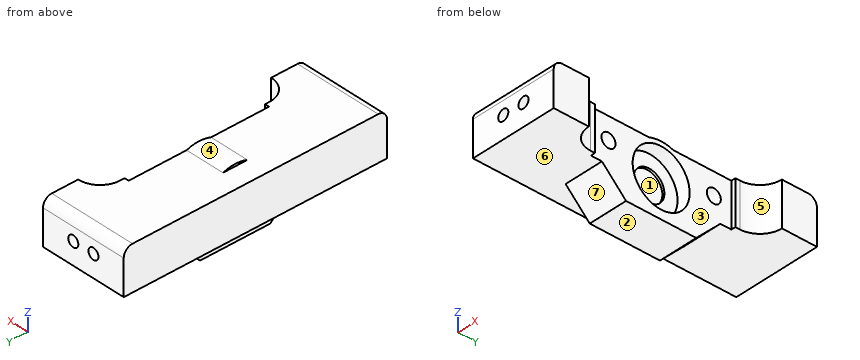
```python
from build123d import *

# Parameters (mm, degrees)
BOX035_W          = 5
BOX035_H          = 60
BOX035_DEPTH      = 10
BOX033_W          = 5
BOX033_H          = 8
BOX033_DEPTH      = 10
FILLET011_R       = 2
BOX034_W          = 5
BOX034_H          = 8
BOX034_DEPTH      = 10
FILLET012_R       = 2
BOX030_W          = 1
BOX030_H          = 32
BOX030_DEPTH      = 22
CYLINDER072_R     = 1.6
CYLINDER072_DEPTH = 10
CYLINDER071_R     = 1.6
CYLINDER071_DEPTH = 10
CYLINDER062_R     = 1.25
CYLINDER062_DEPTH = 10
CYLINDER060_R     = 1.25
CYLINDER060_DEPTH = 10
CYLINDER061_R     = 1.25
CYLINDER061_DEPTH = 10
CYLINDER059_R     = 1.25
CYLINDER059_DEPTH = 10
CYLINDER047_R     = 3.5
CYLINDER047_DEPTH = 4
CYLINDER045_R     = 6.5
CYLINDER045_DEPTH = 4
BOX031_W          = 15
BOX031_H          = 16
BOX031_DEPTH      = 5.5
CYLINDER046_R     = 8
CYLINDER046_DEPTH = 10
BOX021_W          = 10
BOX021_H          = 60
BOX021_DEPTH      = 10
BOX032_W          = 5
BOX032_H          = 60
BOX032_DEPTH      = 10
FILLET010_R       = 2
CHAMFER002_SIZE   = 5.49
FILLET013_R       = 4.99


with BuildPart() as cube014:
    # Box035 → Box035 (new body)
    with BuildSketch(Plane(origin=(75, 1, -1), x_dir=(1, 0, 0), z_dir=(0, 0, 1))):
        with Locations((2.5, 30)):
            Rectangle(BOX035_W, BOX035_H)
    extrude(amount=BOX035_DEPTH)


with BuildPart() as fillet011:
    # Box033 → Box033 (new body)
    with BuildSketch(Plane(origin=(90, 1, 9), x_dir=(1, 0, 0), z_dir=(0, 0, 1))):
        with Locations((2.5, 4)):
            Rectangle(BOX033_W, BOX033_H)
    extrude(amount=BOX033_DEPTH)

    # Fillet011
    fillet011_edges = [fillet011.edges().sort_by_distance(p)[0] for p in [
        (92.5, 1, 19),
    ]]
    fillet(fillet011_edges, radius=FILLET011_R)


with BuildPart() as fillet012:
    # Box034 → Box034 (new body)
    with BuildSketch(Plane(origin=(90, 53, 9), x_dir=(1, 0, 0), z_dir=(0, 0, 1))):
        with Locations((2.5, 4)):
            Rectangle(BOX034_W, BOX034_H)
    extrude(amount=BOX034_DEPTH)

    # Fillet012
    fillet012_edges = [fillet012.edges().sort_by_distance(p)[0] for p in [
        (92.5, 61, 19),
    ]]
    fillet(fillet012_edges, radius=FILLET012_R)


with BuildPart() as cube009:
    # Box030 → Box030 (new body)
    with BuildSketch(Plane(origin=(89, 15, 2), x_dir=(1, 0, 0), z_dir=(0, 0, 1))):
        with Locations((0.5, 16)):
            Rectangle(BOX030_W, BOX030_H)
    extrude(amount=BOX030_DEPTH)


with BuildPart() as cylinder072:
    # Cylinder072 → Cylinder072 (new body)
    with BuildSketch(Plane(origin=(80, 43, 14), x_dir=(0, 0, -1), z_dir=(1, 0, 0))):
        Circle(CYLINDER072_R)
    extrude(amount=CYLINDER072_DEPTH)


with BuildPart() as fusion068:
    # Cylinder071 → Cylinder071 (new body)
    with BuildSketch(Plane(origin=(80, 19, 14), x_dir=(0, 0, -1), z_dir=(1, 0, 0))):
        Circle(CYLINDER071_R)
    extrude(amount=CYLINDER071_DEPTH)

    # Fusion068: union Cylinder072
    add(cylinder072.part)


with BuildPart() as cylinder062:
    # Cylinder062 → Cylinder062 (new body)
    with BuildSketch(Plane(origin=(87.5, 61, 14), x_dir=(1, 0, 0), z_dir=(0, -1, 0))):
        Circle(CYLINDER062_R)
    extrude(amount=CYLINDER062_DEPTH)


with BuildPart() as fusion046:
    # Cylinder060 → Cylinder060 (new body)
    with BuildSketch(Plane(origin=(87.5, 11, 14), x_dir=(1, 0, 0), z_dir=(0, -1, 0))):
        Circle(CYLINDER060_R)
    extrude(amount=CYLINDER060_DEPTH)

    # Fusion046: union Cylinder062
    add(cylinder062.part)


with BuildPart() as cylinder061:
    # Cylinder061 → Cylinder061 (new body)
    with BuildSketch(Plane(origin=(82.5, 61, 14), x_dir=(1, 0, 0), z_dir=(0, -1, 0))):
        Circle(CYLINDER061_R)
    extrude(amount=CYLINDER061_DEPTH)


with BuildPart() as fusion048:
    # Cylinder059 → Cylinder059 (new body)
    with BuildSketch(Plane(origin=(82.5, 11, 14), x_dir=(1, 0, 0), z_dir=(0, -1, 0))):
        Circle(CYLINDER059_R)
    extrude(amount=CYLINDER059_DEPTH)

    # Fusion045: union Cylinder061
    add(cylinder061.part)

    # Fusion048: union Fusion046
    add(fusion046.part)


with BuildPart() as cylinder047:
    # Cylinder047 → Cylinder047 (new body)
    with BuildSketch(Plane(origin=(89.5, 31, 10), x_dir=(0, 0, -1), z_dir=(1, 0, 0))):
        Circle(CYLINDER047_R)
    extrude(amount=CYLINDER047_DEPTH)


with BuildPart() as fusion037:
    # Cylinder045 → Cylinder045 (new body)
    with BuildSketch(Plane(origin=(90, 31, 10), x_dir=(0, 0, -1), z_dir=(1, 0, 0))):
        Circle(CYLINDER045_R)
    extrude(amount=CYLINDER045_DEPTH)

    # Fusion037: union Cylinder047
    add(cylinder047.part)


with BuildPart() as fusion037_1:
    # Fusion037 placement: moved
    add(fusion037.part.moved(Location((-4, 0, 2))))


with BuildPart() as cube010:
    # Box031 → Box031 (new body)
    with BuildSketch(Plane(origin=(75, 23, 3.5), x_dir=(1, 0, 0), z_dir=(0, 0, 1))):
        with Locations((7.5, 8)):
            Rectangle(BOX031_W, BOX031_H)
    extrude(amount=BOX031_DEPTH)


with BuildPart() as cylinder046:
    # Cylinder046 → Cylinder046 (new body)
    with BuildSketch(Plane(origin=(80, 31, 11.5), x_dir=(0, 0, -1), z_dir=(1, 0, 0))):
        Circle(CYLINDER046_R)
    extrude(amount=CYLINDER046_DEPTH)


with BuildPart() as fusion038:
    # Box021 → Box021 (new body)
    with BuildSketch(Plane(origin=(80, 1, 9), x_dir=(1, 0, 0), z_dir=(0, 0, 1))):
        with Locations((5, 30)):
            Rectangle(BOX021_W, BOX021_H)
    extrude(amount=BOX021_DEPTH)

    # Fusion038: union Cylinder046
    add(cylinder046.part)


with BuildPart() as front_threaded_bar_support:
    # Box032 → Box032 (new body)
    with BuildSketch(Plane(origin=(75, 1, 9), x_dir=(1, 0, 0), z_dir=(0, 0, 1))):
        with Locations((2.5, 30)):
            Rectangle(BOX032_W, BOX032_H)
    extrude(amount=BOX032_DEPTH)

    # Fusion069: union Cube010, Fusion038
    add(cube010.part)
    add(fusion038.part)

    # Cut037: cut Fusion037
    add(fusion037_1.part, mode=Mode.SUBTRACT)

    # Cut038: cut Fusion048
    add(fusion048.part, mode=Mode.SUBTRACT)

    # Cut039: cut Fusion068
    add(fusion068.part, mode=Mode.SUBTRACT)

    # Cut040: cut Cube009
    add(cube009.part, mode=Mode.SUBTRACT)

    # Fillet010
    fillet010_edges = [front_threaded_bar_support.edges().sort_by_distance(p)[0] for p in [
        (82.5, 1, 19),
        (82.5, 61, 19),
    ]]
    fillet(fillet010_edges, radius=FILLET010_R)

    # Chamfer002
    chamfer002_edges = [front_threaded_bar_support.edges().sort_by_distance(p)[0] for p in [
        (82, 23, 9),
        (82, 39, 9),
    ]]
    chamfer(chamfer002_edges, length=CHAMFER002_SIZE)

    # Fusion070: union Fillet011, Fillet012
    add(fillet011.part)
    add(fillet012.part)

    # Fillet013
    fillet013_edges = [front_threaded_bar_support.edges().sort_by_distance(p)[0] for p in [
        (90, 53, 14),
        (90, 9, 14),
    ]]
    fillet(fillet013_edges, radius=FILLET013_R)

    # Cut041: cut Cube014
    add(cube014.part, mode=Mode.SUBTRACT)


with BuildPart() as front_threaded_bar_support_1:
    # Cut041 placement: moved
    add(front_threaded_bar_support.part.moved(Location((54, 0, 0))))


solid = front_threaded_bar_support_1.part
```
For this review, take the finished solid that the model builds, in its own axes (mm). Face numbers are marked on the shaded views. A direction names the side the tool comes from. Give positions to 0.01 mm unless a question says otherwise; leave off trailing zeros. Order: outer loops, then holes, each group sorted by start corner. A loop starts at its lowest first (then second) coordinate and runs counter-clockwise, first axis right, second up.
1) Wall thickness on line 1 (Y direction, x = 137.25, z = 14); line 2 (Y direction, x = 138.5, z = 14); line 3 (Y direction, x = 142.35, z = 12): over which ranges is each line inside the solid? List them lowest first.
2) Take a section at C-C (y = 43). Give the boundary of the cut face in (x, z), then the cut area to 3 significant figures.
3) Insertion check: pin 1 (2 mm diameter, centred on y = 31, z = 13, fed in from +X); pin 2 (3.5 mm diameter, centred on y = 43, z = 14, fed in from +X); pin 3 (4 mm diameter, centred on x = 141.5, z = 6.5, fed in from -Y). Each pin has a flat end and moves straight along its axis. Give the tip position at first contact, or say it passes through.
4) Take a section at D-D (z = 7.25). Give the boundary of the cut face in (x, y), then the cut area to 3 significant figures.
5) The part is to be moulded in two halves that separate along Z. For the marked faces 1, 2, 3 and 4, say which applies: released by +Z, released by -Z, zero draft, split by the parting line, or undercut.
6) Take a section at A-A (x = 141.5). State how many separate pieces and enclosed holes the cut face has, then the cut area to 3 significant figures.
7) For the marked faces 5, 6 and 7, list the 3-axis set-ups (+Z, -Z, +X, -X, +Y, -Y) from which the entire face can be reached by the end or side of a thin tool; tool diameter is ignored.
Derived:
1. line 1: y = 11 to 17.4, 20.6 to 41.4, 44.6 to 51
1. line 2: y = 1 to 17.4, 20.6 to 41.4, 44.6 to 61
1. line 3: y = 1 to 24.5, 37.5 to 61
2. outline: (129, 9) - (134, 9) - (134, 7.51) - (143, 7.51) - (143, 12.4) - (134, 12.4) - (134, 15.6) - (143, 15.6) - (143, 19) - (129, 19) - close
2. area: 125 mm2
3. pin 1: stops at x = 139.5
3. pin 2: stops at x = 143
3. pin 3: stops at y = 18.01
4. outline: (134, 19.26) - (143, 19.26) - (143, 26.56) - (140, 26.56) - (140, 35.44) - (143, 35.44) - (143, 42.74) - (134, 42.74) - close
4. area: 185 mm2
5. face 1: undercut
5. face 2: released by -Z
5. face 3: zero draft
5. face 4: released by +Z
6. separate pieces: 1
6. enclosed holes: 3
6. area: 519 mm2
7. face 5: +Z, -Z, +X
7. face 6: -Z, -X
7. face 7: -Z, +X, -X, -Y
